Here's how the part is built. I have some questions about the finished solid (model axes, mm). Coordinates: 2 decimals unless noted, no trailing zeros. Write each loop counter-clockwise with the first axis right and the second up, starting at its lowest first coordinate (ties: lowest second). Pieces come first, ordered by that corner, then holes.
from build123d import *


with BuildPart() as part:
    # Esquisse1 → Base-R_volution (revolve)
    with BuildSketch(Plane.XY, mode=Mode.PRIVATE) as base_r_volution_sk:
        with BuildLine():
            Line((-3.428571429, 6), (3.428571429, 6))
            ThreePointArc((3.428571429, 6), (3.832632446, 6.167367554), (4, 6.571428571))
            Line((4, 6.571428571), (4, 8.285714286))
            Line((4, 8.285714286), (1.511857892, 8.285714286))
            ThreePointArc((1.511857892, 8.285714286), (0, 7.714285714), (-1.511857892, 8.285714286))
            Line((-1.511857892, 8.285714286), (-4, 8.285714286))
            Line((-4, 8.285714286), (-4, 6.571428571))
            ThreePointArc((-4, 6.571428571), (-3.832632446, 6.167367554), (-3.428571429, 6))
        make_face()
    revolve(base_r_volution_sk.sketch.rotate(Axis((0, 0, 0), (1, 0, 0)), 90), axis=Axis((0, 0, 0), (1, 0, 0)))


solid = part.part
1. I want a section at D-D (x = 0.25). List the corners of the cut face in (y, z) for me.
2. For pin 1 Ø3 at (x, z) = (0, 4) entering from -Y; pin 2 Ø2 at (x, y) = (1, 6) entering from -Z, each with a flat end and sliding along its axis, tell me the tip position at first contact or that it passes through.
3. I want a section at A-A (y = 0). List the corners of the cut face in (x, z) for me.
4. If I drill on line 1 (Y direction, x = -1.75, z = 0); line 2 (X direction, y = 6.5, z = 0); line 3 (Z direction, x = 0, y = 5.25), over which ranges is the centre line in solid material (lowest first)?
5. I want a section at C-C (x = 2.5). List the corners of the cut face in (y, z) for me, then the cut area to 3 significant figures.
6. Thinking about a two-plate mould opening in Z: for faces 1 (the face through (-4, -4, -6)), 2 (the face through (0.048, -1.802, 5.723)), 3 (the face through (-2.8, -2.5, 7.9)), which applies, pulls with the +Z half, pulls with the -Z half, needs draft (parallel to the pull), parting line crosses it, or undercut?
Response values:
1. outline: circle Ø15.46 at (0, 0); hole circle Ø12 at (0, 0)
2. pin 1: stops at y = -7.44
2. pin 2: stops at z = -6.5
3. outline: (-4, -8.29) - (-1.51, -8.29) arc R2.29 cw to (1.51, -8.29) - (4, -8.29) - (4, -6.57) arc R0.57 ccw to (3.43, -6) - (-3.43, -6) arc R0.57 ccw to (-4, -6.57) - close; (-4, 6.57) arc R0.57 ccw to (-3.43, 6) - (3.43, 6) arc R0.57 ccw to (4, 6.57) - (4, 8.29) - (1.51, 8.29) arc R2.29 cw to (-1.51, 8.29) - (-4, 8.29) - close
4. line 1: y = -8.29 to -6, 6 to 8.29
4. line 2: x = -4 to 4
4. line 3: z = -5.65 to -2.9, 2.9 to 5.65
5. outline: circle Ø16.57 at (0, 0); hole circle Ø12 at (0, 0)
5. area: 103 mm2
6. face 1: needs draft
6. face 2: undercut
6. face 3: parting line crosses it
